CAD build for the part. Positions are in the model's coordinates, mm. A direction names the side the tool comes from. Coordinates: 2 decimals unless noted, no trailing zeros. Order: outer loops, then holes, each group sorted by start corner. A loop starts at its lowest first (then second) coordinate and runs counter-clockwise, first axis right, second up. Notation, with made-up numbers: M 18,-26 L 32,-26 A29 cw 32,11 Z; hole C 11.5,-37.75 d3. An arc over 180 degrees is marked long. One line per item, written item: value.
from build123d import *

# Parameters (mm, degrees)
SKETCH1_R           = 7.9375
SKETCH1_R_2         = 7.0485
BOSS_EXTRUDE1_DEPTH = 93.93
SKETCH2_R           = 9.525
SKETCH2_R_2         = 7.9375
BOSS_EXTRUDE2_DEPTH = 20
SKETCH3_R           = 8.33501
CUT_EXTRUDE1_DEPTH  = 16.086664195


with BuildPart() as part:
    # Sketch1 → Boss-Extrude1 (new body)
    with BuildSketch(Plane(origin=(0, 0, 0), x_dir=(1, 0, 0), z_dir=(0, 1, 0))):
        with Locations(Location((13.632659162, 6.079429086, 0), (0, 0, 270))):
            Circle(SKETCH1_R)
        with Locations(Location((13.632659162, 6.079429086, 0), (0, 0, 270))):
            Circle(SKETCH1_R_2, mode=Mode.SUBTRACT)
    extrude(amount=BOSS_EXTRUDE1_DEPTH)

    # Sketch2 → Boss-Extrude2 (add)
    with BuildSketch(Plane.XZ):
        with Locations(Location((13.632659162, -6.079429086, 0), (0, 0, 270))):
            Circle(SKETCH2_R)
        with Locations(Location((13.632659162, -6.079429086, 0), (0, 0, 270))):
            Circle(SKETCH2_R_2, mode=Mode.SUBTRACT)
    extrude(amount=-BOSS_EXTRUDE2_DEPTH)

    # Sketch3 → Cut-Extrude1 (cut)
    with BuildSketch(Plane.XZ):
        with Locations(Location((13.632659162, -6.079429086, 0), (0, 0, 270))):
            Circle(SKETCH3_R)
    extrude(amount=-CUT_EXTRUDE1_DEPTH, mode=Mode.SUBTRACT)


solid = part.part
Q1. Mould opens along X. For faces 1 (the face through (6.752, 54.463, -7.607)), 2 (the face through (21.664, 9.86, -11.2)), 3 (the face through (21.44, 20, -3.92)) say: released by +X, released by -X, zero draft, split by the parting line, or undercut.
Recorded:
face 1: undercut
face 2: split by the parting line
face 3: zero draft
Q2. Drill centre lines: line 1 along Y through (x, z) = (11.75, -13); line 2 along Z through (x, y) = (8, 29); line 3 along Z through (x, y) = (15.5, 49). Where is each one in solid material? Low to high.
Recorded:
line 1: y = 16.09 to 93.93
line 2: z = -11.67 to -10.32, -1.84 to -0.49
line 3: z = -13.79 to -12.88, 0.72 to 1.64
Q3. Pin check, flat tips, straight feed: pin 1 Ø8 at (x, y) = (20.5, 56.5) entering from +Z; pin 2 Ø4 at (x, y) = (17.5, 77) entering from -Z; pin 3 Ø1.5 at (x, y) = (17.5, 55) entering from -Z. Stop position of each tip, or through.
Recorded:
pin 1: stops at z = 1.32
pin 2: stops at z = -13.79
pin 3: stops at z = -13.38
Q4. Slice it at D-D (y = 39). List the corners of the cut face in (x, z) (1 decimal), plus the area to 3 significant figures.
Recorded:
outline: C 13.6,-6.1 d15.9; hole C 13.6,-6.1 d14.1
area: 41.9 mm^2
Q5. Which spindle directions (+Z, -Z, +X, -X, +Y, -Y) get a long thin tool onto all of the face, cutting with end or side? Do faces 4 (the face through (20.66, 7.93, -10.56)), 5 (the face through (5.884, 56.447, -7.8)), 6 (the face through (21, 93.93, -6)). Say none if no direction does.
Recorded:
face 4: -Y
face 5: +Y
face 6: +Z, -Z, +X, -X, +Y
Q6. Slice it at C-C (y = 12). List the corners of the cut face in (x, z) (3 decimals).
Recorded:
outline: C 13.633,-6.079 d19.05; hole C 13.633,-6.079 d16.67
Q7. Slice it at A-A (x = 17.75). List the corners of the cut face in (y, z), plus the area to 3 significant figures.
Recorded:
outline: M 0,-14.67 L 20,-14.67 L 20,-12.87 L 93.93,-12.87 L 93.93,-11.8 L 16.09,-11.8 L 16.09,-13.33 L 0,-13.33 Z; M 0,1.17 L 16.09,1.17 L 16.09,-0.36 L 93.93,-0.36 L 93.93,0.71 L 20,0.71 L 20,2.51 L 0,2.51 Z
area: 223 mm^2
Q8. Slice it at B-B (z = -1.25). List the corners of the cut face in (x, y).
Recorded:
outline: M 5.42,0 L 6.84,0 L 6.84,16.09 L 8.5,16.09 L 8.5,93.93 L 7.33,93.93 L 7.33,20 L 5.42,20 Z; M 18.77,16.09 L 20.43,16.09 L 20.43,0 L 21.84,0 L 21.84,20 L 19.93,20 L 19.93,93.93 L 18.77,93.93 Z
